Geometry check sheet. Reference: the model listing, model coordinates, mm. Face numbers are marked on the shaded views. Round coordinates to 2 decimals unless told otherwise and drop trailing zeros. Write each loop counter-clockwise with the first axis right and the second up, starting at its lowest first coordinate (ties: lowest second). Pieces come first, ordered by that corner, then holes. Notation, with made-up numbers: (-24, -36) -> (33, -36) arc R13 ccw to (33, -30) -> close; hole circle Ø5 at (58.25, 66.25). An arc over 180 degrees is marked (long way). Return JSON: item names as keys, results as strings. Group by question number.
from build123d import *

# Parameters (mm, degrees)
SKETCH1_W           = 62
SKETCH1_H           = 60
BOSS_EXTRUDE1_DEPTH = 2
SKETCH2_W           = 2
SKETCH2_H           = 59.995898743
BOSS_EXTRUDE2_DEPTH = 30
FILLET1_R           = 1
SKETCH3_R           = 19
CUT_EXTRUDE1_DEPTH  = 54.712196008


with BuildPart() as part:
    # Sketch1 → Boss-Extrude1 (new body)
    with BuildSketch(Plane(origin=(0, 0, 0), x_dir=(1, 0, 0), z_dir=(0, 1, 0))):
        Rectangle(SKETCH1_W, SKETCH1_H)
    extrude(amount=BOSS_EXTRUDE1_DEPTH)

    # Sketch2 → Boss-Extrude2 (add)
    with BuildSketch(Plane.XZ):
        with Locations((-30, 0.002050629)):
            Rectangle(SKETCH2_W, SKETCH2_H)
    extrude(amount=BOSS_EXTRUDE2_DEPTH)

    # Fillet1
    fillet1_edges = [part.edges().sort_by_distance(p)[0] for p in [
        (-31, 2, 0),
        (-29, 0, 0.002050628),
    ]]
    fillet(fillet1_edges, radius=FILLET1_R)

    # Sketch3 → Cut-Extrude1 (cut, through all)
    with BuildSketch(Plane(origin=(0, 2, 0), x_dir=(1, 0, 0), z_dir=(0, 1, 0))):
        with Locations(Location((0, 0, 0), (0, 0, 270))):
            Circle(SKETCH3_R)
    extrude(amount=-CUT_EXTRUDE1_DEPTH, mode=Mode.SUBTRACT)


solid = part.part
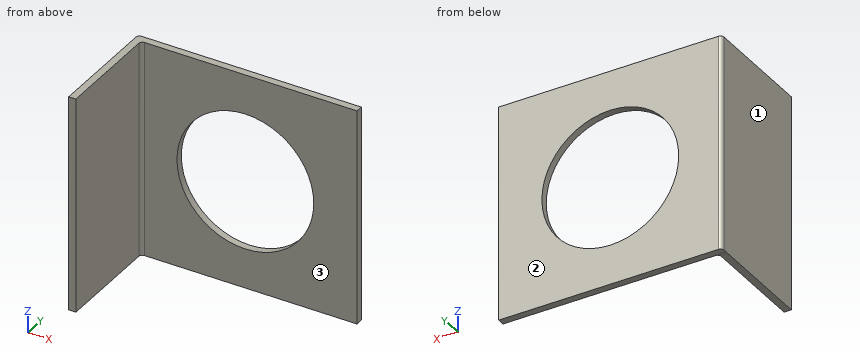
1) Mould release check, pull along Y, two halves, no side actions. Record for the marked faces 1, 2 and 3: +Y half, -Y half, draft (parallel to the pull), parting line (faces both ways), or undercut.
2) Sectioned sample at A-A on x = 0. Enter the section's corners in (y, z).
3) Sectioned sample at C-C on y = -16. Enter the section's corners in (x, z).
4) Go/stop test with flat-tipped pins: P1, Ø1, axis at y = -26, z = -15, coming from the +X side; P2, Ø2, axis at x = -10.5, z = -21.5, coming from the -Y side; P3, Ø2.5, axis at x = -30, y = -10, coming from the -Z side. Record where each tip stops, or that it passes through.
5) Sectioned sample at B-B on z = 0. Enter the section's corners in (x, y).
6) Sectioned sample at D-D on x = 14. Enter the section's corners in (y, z).
7) Material ranges on probe 1 along X at (y, z) = (-26.5, -16.5); probe 2 along Y at (x, z) = (-25, -22), recorded low to high. Write a range as [from, to].
Evaluation:
{
 "1": {"face 1": "draft", "face 2": "+Y half", "face 3": "-Y half"},
 "2": {"outline": "(0, -30) -> (2, -30) -> (2, -19) -> (0, -19) -> close; (0, 19) -> (2, 19) -> (2, 30) -> (0, 30) -> close"},
 "3": {"outline": "(-31, -30) -> (-29, -30) -> (-29, 30) -> (-31, 30) -> close"},
 "4": {"P1": "stops at x = -29", "P2": "stops at y = 0", "P3": "stops at z = -30"},
 "5": {"outline": "(-31, -30) -> (-29, -30) -> (-29, -1) arc R1 cw to (-28, 0) -> (-19, 0) -> (-19, 2) -> (-30, 2) arc R1 ccw to (-31, 1) -> close; (19, 0) -> (31, 0) -> (31, 2) -> (19, 2) -> close"},
 "6": {"outline": "(0, -30) -> (2, -30) -> (2, -12.85) -> (0, -12.85) -> close; (0, 12.85) -> (2, 12.85) -> (2, 30) -> (0, 30) -> close"},
 "7": {"probe 1": "x = [-31, -29]", "probe 2": "y = [0, 2]"}
}
